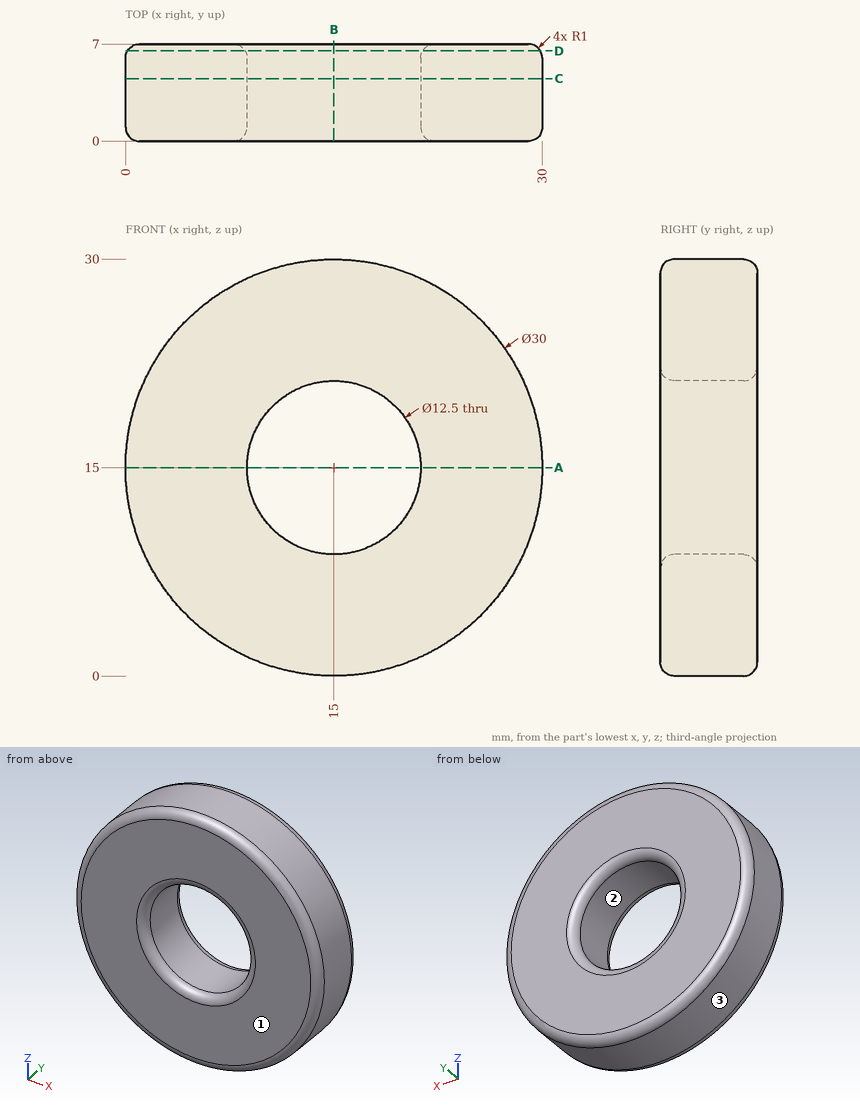
Here's the drawing with two shaded views (mm, measured from the low corner). I have some questions. Round coordinates to 2 decimals unless told otherwise and drop trailing zeros. Order: outer loops, then holes, each group sorted by start corner. A loop starts at its lowest first (then second) coordinate and runs counter-clockwise, first axis right, second up. Notation, with made-up numbers: (-3, 30.5) -> (35, 30.5) arc R20 ccw to (35, 66.5) -> close; hole circle Ø4 at (-34, -23.75). An arc over 180 degrees is marked (long way). Return JSON: item names as keys, results as strings.
Q1. If we section it at B-B on x = 15: List the corners of the cut face in (y, z) for me, plus the area to 3 significant figures.
Filled sheet:
{"outline": "(0, 1) arc R1 ccw to (1, 0) -> (6, 0) arc R1 ccw to (7, 1) -> (7, 7.75) arc R1 ccw to (6, 8.75) -> (1, 8.75) arc R1 ccw to (0, 7.75) -> close; (0, 22.25) arc R1 ccw to (1, 21.25) -> (6, 21.25) arc R1 ccw to (7, 22.25) -> (7, 29) arc R1 ccw to (6, 30) -> (1, 30) arc R1 ccw to (0, 29) -> close", "area": "121 mm^2"}
Q2. I need wall thicknesses on line 1 along Z through (x, y) = (15.25, 6) (3 decimals); line 2 along Z through (x, y) = (9.25, 4); line 3 along X through (y, z) = (4.5, 19.5). Which ranges of each line are inside material? Lowest first, please. Write a range as from..to.
Filled sheet:
{"line 1": "z = 0.002..8.755, 21.245..29.998", "line 2": "z = 1.15..12.55, 17.45..28.85", "line 3": "x = 0.69..10.66, 19.34..29.31"}
Q3. If we section it at A-A on z = 15: List the corners of the cut face in (x, y) for me.
Filled sheet:
{"outline": "(0, 1) arc R1 ccw to (1, 0) -> (7.75, 0) arc R1 ccw to (8.75, 1) -> (8.75, 6) arc R1 ccw to (7.75, 7) -> (1, 7) arc R1 ccw to (0, 6) -> close; (21.25, 1) arc R1 ccw to (22.25, 0) -> (29, 0) arc R1 ccw to (30, 1) -> (30, 6) arc R1 ccw to (29, 7) -> (22.25, 7) arc R1 ccw to (21.25, 6) -> close"}
Q4. If we section it at C-C on y = 4.5: List the corners of the cut face in (x, z) for me.
Filled sheet:
{"outline": "circle Ø30 at (15, 15); hole circle Ø12.5 at (15, 15)"}
Q5. If we mould it in two halves opening along X, with no side actions, what happens to the marked faces 1, 2 and 3? For each: released by +X, released by -X, zero draft, split by the parting line, or undercut.
Filled sheet:
{"face 1": "zero draft", "face 2": "undercut", "face 3": "split by the parting line"}
Q6. If we section it at D-D on y = 6.5: List the corners of the cut face in (x, z) for me, plus the area to 3 significant figures.
Filled sheet:
{"outline": "circle Ø29.73 at (15, 15); hole circle Ø12.77 at (15, 15)", "area": "566 mm^2"}
Q7. For pin 1 Ø1.5 at (y, z) = (1, 3) entering from -X; pin 2 Ø2 at (y, z) = (6, 24.5) entering from -X, each with a flat end and sliding along its axis, tell me the tip position at first contact or that it passes through.
Filled sheet:
{"pin 1": "stops at x = 5.08", "pin 2": "stops at x = 2.64"}
